Check sheet for the modelled part. Datum: model origin and axes. Units: mm. Face numbers are marked on the shaded views. Round coordinates to 2 decimals unless told otherwise and drop trailing zeros. Write each loop counter-clockwise with the first axis right and the second up, starting at its lowest first coordinate (ties: lowest second). Pieces come first, ordered by that corner, then holes. Notation, with made-up numbers: (17, 70.25) - (69, 70.25) arc R29 cw to (69, 109.25) - close; hole circle Ø7 at (17.25, -5). An arc over 180 degrees is marked (long way). Use one line per item in the form item = value. Start each with the question number.
1) Section check B-B (z = 0). Record the boundary of the cut face in (x, y), then the cut area to 3 significant figures.
2) Scan lines: probe 1 along Z at (x, y) = (-32, 2.2); probe 2 along Z at (x, y) = (-32, 2.85); probe 3 along X at (y, z) = (1, 0). Record each from-to range of solid material in increasing order.
3) Gauge pin test, flat ends, axial feed: P1, Ø8.5, axis at x = 32, z = 32, coming from the +Y side; P2, Ø1.5, axis at x = -13, z = -10.5, coming from the +Y side; P3, Ø6, axis at y = 6, z = -28, coming from the -X side. Record the tip position at first contact, or that the pin passes through.
4) Section check D-D (x = 34). Count the separate pieces of the cut face and the enclosed holes in it, then the cut area to 3 significant figures.
5) Section check A-A (x = 0). Record the boundary of the cut face in (y, z).
6) Draft check along X on the marked faces 1 and 2. Enter one of: +X half, -X half, draft (parallel to the pull), parting line (faces both ways), or undercut.
7) Section check C-C (y = 6). Record the boundary of the cut face in (x, z), then the cut area to 3 significant figures.
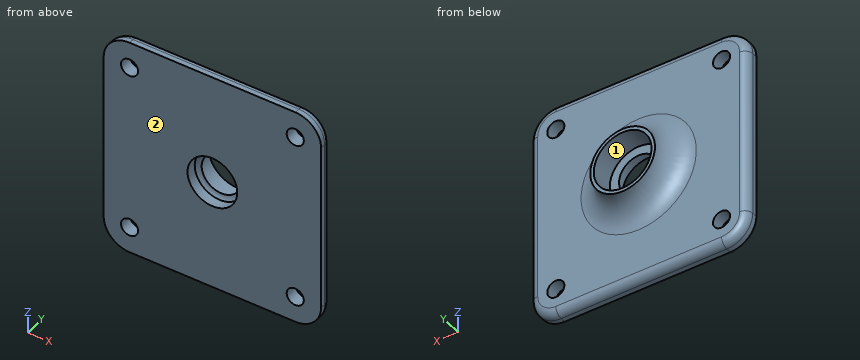
from build123d import *

# Parameters (mm, degrees)
BOSS_EXTRUDE1_DEPTH      = 5
FILLET1_R                = 3
M6_CLEARANCE_HOLE1_D     = 6.6
M6_CLEARANCE_HOLE1_DEPTH = 8
M6_CLEARANCE_HOLE1_TIP   = 1.982840043


with BuildPart() as part:
    # Sketch1 → Boss-Extrude1 (new body)
    with BuildSketch(Plane(origin=(0, 0, 0), x_dir=(1, 0, 0), z_dir=(0, 1, 0))):
        with BuildLine():
            Line((32, 42), (-32, 42))
            ThreePointArc((-32, 42), (-39.071067812, 39.071067812), (-42, 32))
            Line((-42, 32), (-42, -32))
            ThreePointArc((-42, -32), (-39.071067812, -39.071067812), (-32, -42))
            Line((-32, -42), (32, -42))
            ThreePointArc((32, -42), (39.071067812, -39.071067812), (42, -32))
            Line((42, -32), (42, 32))
            ThreePointArc((42, 32), (39.071067812, 39.071067812), (32, 42))
        make_face()
    extrude(amount=BOSS_EXTRUDE1_DEPTH)

    # Sketch3 → Revolve2 (revolve)
    with BuildSketch(Plane.XY, mode=Mode.PRIVATE) as revolve2_sk:
        with BuildLine():
            Line((-22.25, 5), (-12.5, 5))
            Line((-12.5, 5), (-11.15, 5))
            Line((-11.15, 5), (-11.15, 14))
            Line((-11.15, 14), (-12.5, 14))
            ThreePointArc((-12.5, 14), (-15.66727432, 7.649963846), (-22.25, 5))
        make_face()
    revolve(revolve2_sk.sketch.rotate(Axis((0, 0, 0), (0, -1, 0)), 270), axis=Axis((0, 0, 0), (0, -1, 0)))

    # Sketch3_5 → Cut-Revolve2 (revolve, cut)
    with BuildSketch(Plane.XY, mode=Mode.PRIVATE) as cut_revolve2_sk:
        with BuildLine():
            Line((0, 0), (0, 5))
            Line((0, 5), (-7.6, 5))
            ThreePointArc((-7.6, 5), (-8.694616444, 4.701278719), (-9.6, 4.017392631))
            Line((-9.6, 4.017392631), (-9.6, 0))
            Line((-9.6, 0), (0, 0))
        make_face()
    revolve(cut_revolve2_sk.sketch.rotate(Axis((0, 0, 0), (0, -1, 0)), 270), axis=Axis((0, 0, 0), (0, -1, 0)), mode=Mode.SUBTRACT)

    # Fillet1
    fillet1_edges = [part.edges().sort_by_distance(p)[0] for p in [
        (39.071067812, 5, 39.071067812),
        (0, 5, 42),
        (-39.071067812, 5, 39.071067812),
        (-42, 5, 0),
        (-39.071067812, 5, -39.071067812),
        (0, 5, -42),
        (39.071067812, 5, -39.071067812),
        (42, 5, 0),
    ]]
    fillet(fillet1_edges, radius=FILLET1_R)

    # M6 Clearance Hole1
    with Locations(Plane(origin=(0, 5, 0), x_dir=(1, 0, 0), z_dir=(0, 1, 0))):
        with Locations((-32, 32), (-32, -32), (32, -32), (32, 32)):
            Hole(M6_CLEARANCE_HOLE1_D / 2, depth=M6_CLEARANCE_HOLE1_DEPTH)
            with Locations((0, 0, -(M6_CLEARANCE_HOLE1_DEPTH + M6_CLEARANCE_HOLE1_TIP / 2))):  # 118° drill point
                Cone(0, M6_CLEARANCE_HOLE1_D / 2, M6_CLEARANCE_HOLE1_TIP, mode=Mode.SUBTRACT)


solid = part.part
Results are:
q1.outline = (-42, 0) - (-9.6, 0) - (-9.6, 4.02) arc R3 cw to (-7.6, 5) - (-11.15, 5) - (-11.15, 14) - (-12.5, 14) arc R10 cw to (-22.25, 5) - (-39, 5) arc R3 ccw to (-42, 2) - close; (7.6, 5) arc R3 cw to (9.6, 4.02) - (9.6, 0) - (42, 0) - (42, 2) arc R3 ccw to (39, 5) - (22.25, 5) arc R10 cw to (12.5, 14) - (11.15, 14) - (11.15, 5) - close
q1.area = 388 mm²
q2.probe_1 = -41.99 to -35.3, -28.7 to 28.7, 35.3 to 41.99
q2.probe_2 = -41.88 to -35.3, -28.7 to 28.7, 35.3 to 41.88
q2.probe_3 = -42 to -9.6, 9.6 to 42
q3.P1 = 5
q3.P2 = 7.39
q3.P3 = -41.83
q4.separate_pieces = 3
q4.enclosed_holes = 0
q4.area = 362 mm²
q5.outline = (0, -42) - (2, -42) arc R3 ccw to (5, -39) - (5, -22.25) arc R10 cw to (14, -12.5) - (14, -11.15) - (5, -11.15) - (5, -7.6) arc R3 cw to (4.02, -9.6) - (0, -9.6) - close; (0, 9.6) - (4.02, 9.6) arc R3 cw to (5, 7.6) - (5, 11.15) - (14, 11.15) - (14, 12.5) arc R10 cw to (5, 22.25) - (5, 39) arc R3 ccw to (2, 42) - (0, 42) - close
q6.face_1 = undercut
q6.face_2 = draft
q7.outline = circle Ø36.17 at (0, 0); hole circle Ø22.3 at (0, 0)
q7.area = 637 mm²
